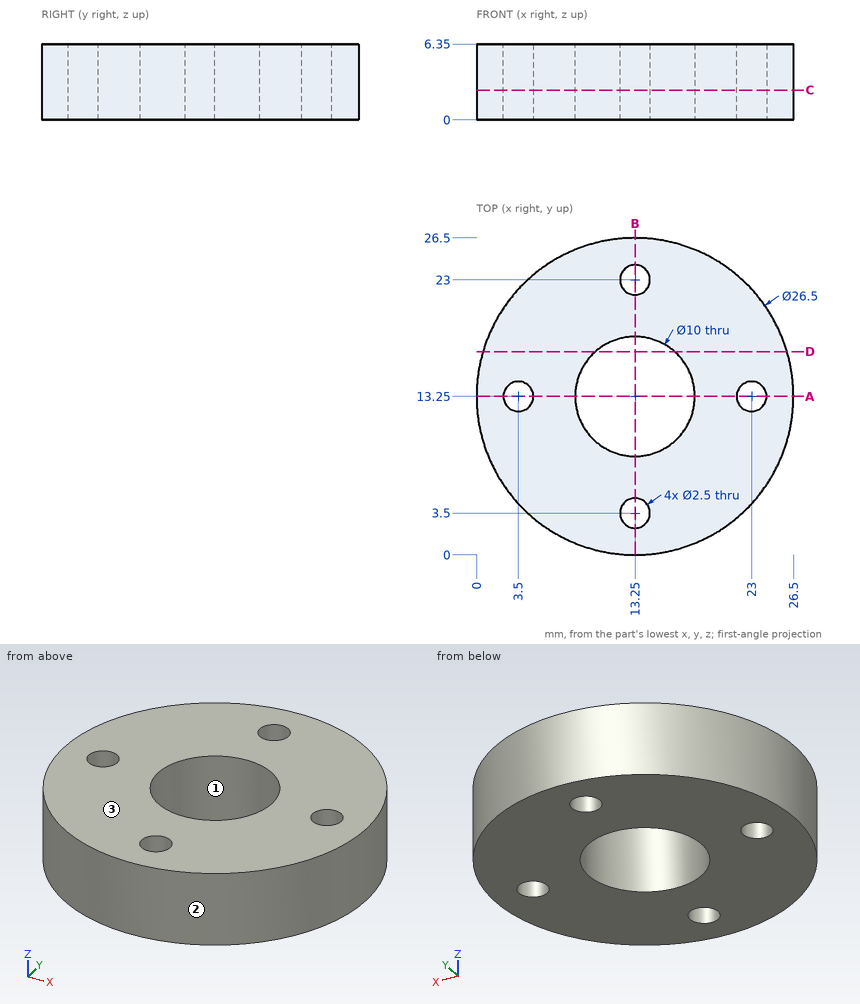
Check sheet for the drawn part. Datum: minimum x, y, z corner. Units: mm. Round coordinates to 2 decimals unless told otherwise and drop trailing zeros. Write each loop counter-clockwise with the first axis right and the second up, starting at its lowest first coordinate (ties: lowest second). Pieces come first, ordered by that corner, then holes. Notation, with made-up numbers: (27.25, 23) -> (53.25, 23) arc R16 ccw to (53.25, 41) -> close; hole circle Ø6 at (3.5, 58.5). An arc over 180 degrees is marked (long way). One line per item, written item: value. Start each with the question number.
(1) Cross-section at C-C, the plane z = 2.5. Record the cut outline in (x, y), and give its area (3 significant figures).
(2) Cross-section at D-D, the plane y = 17. Record the cut outline in (x, z).
(3) Go/stop test with flat-tipped pins: pin 1 Ø3 at (y, z) = (9.5, 5) entering from -X; pin 2 Ø2 at (y, z) = (15.5, 1.5) entering from -X; pin 3 Ø1.5 at (x, y) = (3.5, 13.25) entering from +Z (1 decimal); pin 4 Ø6 at (x, y) = (23.5, 6.5) entering from -Z. Record where each tip stops, or that it passes through.
(4) Draft check along X on the marked faces 1, 2 and 3. Enter one of: +X half, -X half, draft (parallel to the pull), parting line (faces both ways), or undercut.
(5) Cross-section at A-A, the plane y = 13.25. Record the cut outline in (x, z).
(6) Scan lines: line 1 (Y direction, x = 13.25, z = 5); line 2 (X direction, y = 12.25, z = 3.5); line 3 (X direction, y = 13.75, z = 3.5). Record each from-to range of solid material in increasing order. Write a range as [from, to].
Answer:
1. outline: circle Ø26.5 at (13.25, 13.25); hole circle Ø2.5 at (3.5, 13.25); hole circle Ø10 at (13.25, 13.25); hole circle Ø2.5 at (13.25, 3.5); hole circle Ø2.5 at (13.25, 23); hole circle Ø2.5 at (23, 13.25)
1. area: 453 mm²
2. outline: (0.54, 0) -> (9.94, 0) -> (9.94, 6.35) -> (0.54, 6.35) -> close; (16.56, 0) -> (25.96, 0) -> (25.96, 6.35) -> (16.56, 6.35) -> close
3. pin 1: x = 0.19
3. pin 2: x = 0.06
3. pin 3: through
3. pin 4: z = 0
4. face 1: undercut
4. face 2: parting line
4. face 3: draft
5. outline: (0, 0) -> (2.25, 0) -> (2.25, 6.35) -> (0, 6.35) -> close; (4.75, 0) -> (8.25, 0) -> (8.25, 6.35) -> (4.75, 6.35) -> close; (18.25, 0) -> (21.75, 0) -> (21.75, 6.35) -> (18.25, 6.35) -> close; (24.25, 0) -> (26.5, 0) -> (26.5, 6.35) -> (24.25, 6.35) -> close
6. line 1: [0, 2.25], [4.75, 8.25], [18.25, 21.75], [24.25, 26.5]
6. line 2: [0.04, 2.75], [4.25, 8.35], [18.15, 22.25], [23.75, 26.46]
6. line 3: [0.01, 2.35], [4.65, 8.28], [18.22, 21.85], [24.15, 26.49]
